```python
from build123d import *

# Parameters (mm, degrees)
SKETCH2_W           = 10
SKETCH2_H           = 20
BOSS_EXTRUDE1_DEPTH = 15
SKETCH3_W           = 4.1
SKETCH3_H           = 15.1
CUT_EXTRUDE1_DEPTH  = 16
SKETCH4_W           = 2.95
SKETCH4_H           = 2.45
CUT_EXTRUDE2_DEPTH  = 15
SKETCH6_W           = 20
SKETCH6_H           = 15
BOSS_EXTRUDE2_DEPTH = 3
BOSS_EXTRUDE3_DEPTH = 5
CUT_EXTRUDE3_DEPTH  = 21
CUT_EXTRUDE4_DEPTH  = 0.5


with BuildPart() as part:
    # Sketch2 → Boss-Extrude1 (new body)
    with BuildSketch(Plane(origin=(0, 0, 0), x_dir=(1, 0, 0), z_dir=(0, 1, 0))):
        Rectangle(SKETCH2_W, SKETCH2_H)
    extrude(amount=BOSS_EXTRUDE1_DEPTH)

    # Sketch3 → Cut-Extrude1 (cut, through all)
    with BuildSketch(Plane(origin=(0, 15, 0), x_dir=(1, 0, 0), z_dir=(0, 1, 0))):
        Rectangle(SKETCH3_W, SKETCH3_H)
    extrude(amount=-CUT_EXTRUDE1_DEPTH, mode=Mode.SUBTRACT)

    # Sketch4 → Cut-Extrude2 (cut)
    with BuildSketch(Plane(origin=(0, 15, 0), x_dir=(1, 0, 0), z_dir=(0, 1, 0))):
        Polygon((-2.05, 10), (-5, 10), (-5, -7.55), (-2.05, -7.55), (-2.05, 7.55), align=None)
        with Locations((-3.525, -8.775)):
            Rectangle(SKETCH4_W, SKETCH4_H)
    extrude(amount=-CUT_EXTRUDE2_DEPTH, mode=Mode.SUBTRACT)

    # Sketch6 → Boss-Extrude2 (add)
    with BuildSketch(Plane.ZY.offset(2.05)):
        with Locations((0, 7.5)):
            Rectangle(SKETCH6_W, SKETCH6_H)
    extrude(amount=BOSS_EXTRUDE2_DEPTH)

    # Sketch8 → Boss-Extrude3 (add)
    with BuildSketch(Plane.ZY.offset(5.05)):
        Polygon((-7, 15), (-10, 15), (-10, 0), (10, 0), (10, 15), (7, 15), (7, 3), (-7, 3), align=None)
    extrude(amount=BOSS_EXTRUDE3_DEPTH)

    # Sketch10 → Cut-Extrude3 (cut, through all)
    with BuildSketch(Plane.XY.offset(10)):
        Polygon((-10.05, 0), (5, 8.689121551), (5, 0), align=None)
    extrude(amount=-CUT_EXTRUDE3_DEPTH, mode=Mode.SUBTRACT)

    # Sketch11 → Cut-Extrude4 (cut)
    with BuildSketch(Plane.ZY.offset(10.05)):
        Polygon((-8, 2), (-8, 15), (-9, 15), (-9, 1), (0, 1), (9, 1), (9, 15), (8, 15), (8, 2), (0, 2), align=None)
    extrude(amount=-CUT_EXTRUDE4_DEPTH, mode=Mode.SUBTRACT)


solid = part.part
```
Can you work these out from the model? Positions are in its coordinate system, mm. A direction names the side the tool comes from. Coordinates: 2 decimals unless noted, no trailing zeros. Loops run counter-clockwise (first coordinate to the right, second up) from the corner with the lowest first, then second, coordinate; pieces in that order, holes last. Notation, with made-up numbers: (-17.75, 34.5) -> (-5.75, 34.5) arc R27 cw to (-5.75, 71.5) -> close; hole circle Ø10 at (-21, 21.25). An arc over 180 degrees is marked (long way). Answer as a JSON object with one key per item and string values.
1) For P1, Ø5.5, axis at x = -7, z = 2.5, coming from the +Y side; P2, Ø3, axis at y = 7, z = -5, coming from the +X side; P3, Ø7, axis at y = 10, z = 1.5, coming from the -X side; P4, Ø8, axis at x = -3, z = 1.5, coming from the -Y side, each with a flat end and sliding along its axis, tell me the tip position at first contact or that it passes through.
Results:
{"P1": "stops at y = 15", "P2": "stops at x = 4.67", "P3": "stops at x = -5.05", "P4": "stops at y = 1.76"}
2) Imagine slicing it at D-D (z = -8.5). Please give me the cut outline in (x, y).
Results:
{"outline": "(-10.05, 0) -> (5, 8.69) -> (5, 15) -> (-9.55, 15) -> (-9.55, 1) -> (-10.05, 1) -> close"}
3) If I drill on line 1 (Z direction, x = -2, y = 14); line 2 (X direction, y = 10, z = 3.25); line 3 (Z direction, x = -8, y = 8.75), over which ranges is the centre line in solid material (lowest first)?
Results:
{"line 1": "z = -10 to -7.55, 7.55 to 10", "line 2": "x = -5.05 to -2.05, 2.05 to 5", "line 3": "z = -10 to -7, 7 to 10"}
4) Imagine slicing it at B-B (x = 1). Please give me the cut outline in (y, z).
Results:
{"outline": "(6.38, -10) -> (15, -10) -> (15, -7.55) -> (6.38, -7.55) -> close; (6.38, 7.55) -> (15, 7.55) -> (15, 10) -> (6.38, 10) -> close"}
5) Imagine slicing it at C-C (y = 10.5). Please give me the cut outline in (x, z).
Results:
{"outline": "(-10.05, -10) -> (5, -10) -> (5, 10) -> (-10.05, 10) -> (-10.05, 9) -> (-9.55, 9) -> (-9.55, 8) -> (-10.05, 8) -> (-10.05, 7) -> (-5.05, 7) -> (-5.05, -7) -> (-10.05, -7) -> (-10.05, -8) -> (-9.55, -8) -> (-9.55, -9) -> (-10.05, -9) -> close; hole (-2.05, -7.55) -> (2.05, -7.55) -> (2.05, 7.55) -> (-2.05, 7.55) -> close"}
6) Thinking about a two-plate mould opening in Y: for faces 4 (the face through (-2.6, 4.3, 0.1)), 5 (the face through (2.05, 11, 0)), 6 (the face through (-9.55, 1.8, -1.4)), which applies, pulls with the +Y half, pulls with the -Y half, needs draft (parallel to the pull), parting line crosses it, or undercut?
Results:
{"face 4": "pulls with the -Y half", "face 5": "needs draft", "face 6": "undercut"}
7) For faces 1 (the face through (-2.4, 15, 0.1)), 2 (the face through (-2.05, 10, 0)), 3 (the face through (-8, 3, 0)), which set-ups out of +Z, -Z, +X, -X, +Y, -Y let a thin tool reach every point of the face, with its end or its side?
Results:
{"face 1": "+Z, -Z, +X, -X, +Y", "face 2": "+Y, -Y", "face 3": "-X, +Y"}
8) Imagine slicing it at A-A (z = 3.75). Please give me the cut outline in (x, y), then the cut area to 3 significant figures.
Results:
{"outline": "(-10.05, 0) -> (-2.05, 4.62) -> (-2.05, 15) -> (-5.05, 15) -> (-5.05, 3) -> (-10.05, 3) -> (-10.05, 2) -> (-9.55, 2) -> (-9.55, 1) -> (-10.05, 1) -> close; (2.05, 6.99) -> (5, 8.69) -> (5, 15) -> (2.05, 15) -> close", "area": "62.2 mm^2"}
